Work out the finished part from the listing and answer in its coordinate system (mm). A direction names the side the tool comes from. Coordinates: 2 decimals unless noted, no trailing zeros. Order: outer loops, then holes, each group sorted by start corner. A loop starts at its lowest first (then second) coordinate and runs counter-clockwise, first axis right, second up.
1. Flat-ended cylindrical pins translate along their axes: pin 1 Ø1 at (x, z) = (-2.5, 23) entering from -Y; pin 2 Ø0.5 at (y, z) = (-2, 0) entering from -X; pin 3 Ø0.5 at (y, z) = (-1.5, 2) entering from +X. Find the tip coordinate at first contact, or state that the pin passes through.
2. Find the intervals of material crossed by probe 1 along X at (y, z) = (-1.75, 2); probe 2 along Z at (x, y) = (11.25, -1.8); probe 3 along X at (y, z) = (-2.4, 26.5), in increasing order.
3. A tool of negligible diameter and unlimited length cuts with its end or side. For faces 1 (the flat face through (2.54, -2, 1)), 2 (the cylindrical face through (7.07, -2.819, 5.405)), from which of +Z, -Z, +X, -X, +Y, -Y can it reach the whole face along a straight path? Write none if from no direction.
4. The part is cut by section A-A, the plane y = -1.6. Give the vertices of the cut face in (x, z), then the cut area to 3 significant figures.
```python
from build123d import *

# Parameters (mm, degrees)
F1_DEPTH = 3.048
F2_R     = 0.762


with BuildPart() as f1:
    # F0 (on Front) → F1 (new body)
    with BuildSketch(Plane.XZ):
        Polygon((0, 31.242), (-5.842, 13.187891), (-12.7, 9.228423), (-12.7, 6.688423), (-2.54, 3.966059), (-2.54, -1.875941), (2.54, -1.875941), (2.54, 3.966059), (12.7, 6.688423), (12.7, 9.228423), (5.842, 13.187891), align=None)
    extrude(amount=F1_DEPTH)

    # F2
    f2_edges = [f1.edges().sort_by_distance(p)[0] for p in [
        (0, -1.524, 31.242),
        (5.842, -1.524, 13.187891),
        (12.7, -1.524, 9.228423),
        (12.7, -1.524, 6.688423),
        (-5.842, -1.524, 13.187891),
        (-12.7, -1.524, 9.228423),
        (-12.7, -1.524, 6.688423),
        (2.54, 0, 1.045059),
        (2.54, -3.048, 1.045059),
        (-2.54, -3.048, 1.045059),
        (-2.54, 0, 1.045059),
        (2.921, -3.048, 22.214946),
        (-2.921, -3.048, 22.214946),
        (-9.271, -3.048, 11.208157),
        (-12.7, -3.048, 7.958423),
        (-7.62, -3.048, 5.327241),
        (0, -3.048, -1.875941),
        (7.62, -3.048, 5.327241),
        (12.7, -3.048, 7.958423),
        (9.271, -3.048, 11.208157),
        (2.921, 0, 22.214946),
        (-2.921, 0, 22.214946),
        (-9.271, 0, 11.208157),
        (-12.7, 0, 7.958423),
        (-7.62, 0, 5.327241),
        (0, 0, -1.875941),
        (7.62, 0, 5.327241),
        (12.7, 0, 7.958423),
        (9.271, 0, 11.208157),
    ]]
    fillet(f2_edges, radius=F2_R)


solid = f1.part
```
Geometry says:
1. pin 1: stops at y = -3.04
1. pin 2: stops at x = -2.54
1. pin 3: stops at x = 2.54
2. probe 1: x = -2.54 to 2.54
2. probe 2: z = 6.3 to 10.07
2. probe 3: x = -1.53 to 1.53
3. face 1: -Z, +X, +Y, -Y
3. face 2: -Z, +X, -Y
4. outline: (-12.7, 7.27) arc R0.76 ccw to (-12.14, 6.54) - (-2.54, 3.97) - (-2.54, -1.88) - (2.54, -1.88) - (2.54, 3.97) - (12.14, 6.54) arc R0.76 ccw to (12.7, 7.27) - (12.7, 8.79) arc R0.76 ccw to (12.32, 9.45) - (6.1, 13.04) arc R0.76 cw to (5.75, 13.47) - (0.72, 29) arc R0.76 ccw to (-0.72, 29) - (-5.75, 13.47) arc R0.76 cw to (-6.1, 13.04) - (-12.32, 9.45) arc R0.76 ccw to (-12.7, 8.79) - close
4. area: 313 mm2
